Verification items for the finished model (mm, model axes). A direction names the side the tool comes from. Give positions to 0.01 mm unless a question says otherwise; leave off trailing zeros. Loops run counter-clockwise (first coordinate to the right, second up) from the corner with the lowest first, then second, coordinate; pieces in that order, holes last. Notation, with made-up numbers: (36.5, 41.5) - (55.5, 41.5) arc R25 ccw to (55.5, 65.5) - close; hole circle Ø8 at (22.25, -6). An arc over 180 degrees is marked (long way). Answer in a Markdown table with one row per item.
```python
from build123d import *

# Parameters (mm, degrees)
ESQUISSE1_R        = 1.6
BOSS_EXTRU_1_DEPTH = 1.6
ESQUISSE2_W        = 11
ESQUISSE2_H        = 9
BOSS_EXTRU_2_DEPTH = 12.7
ESQUISSE3_W        = 32.2
ESQUISSE3_H        = 9.1
BOSS_EXTRU_3_DEPTH = 14.9
ESQUISSE4_W        = 35.56
ESQUISSE4_H        = 17.78
BOSS_EXTRU_4_DEPTH = 12


with BuildPart() as part:
    # Esquisse1 → Boss.-Extru.1 (new body)
    with BuildSketch(Plane.XY):
        Polygon((0, 0), (100, 0), (100, -70), (30, -70), (0, -40), align=None)
        with Locations((3.5, -3.5)):
            Circle(ESQUISSE1_R, mode=Mode.SUBTRACT)
        with Locations((96.5, -3.5)):
            Circle(ESQUISSE1_R, mode=Mode.SUBTRACT)
        with Locations((3.5, -38.5)):
            Circle(ESQUISSE1_R, mode=Mode.SUBTRACT)
        with Locations((96.5, -66.5)):
            Circle(ESQUISSE1_R, mode=Mode.SUBTRACT)
    extrude(amount=BOSS_EXTRU_1_DEPTH)

    # Esquisse2 → Boss.-Extru.2 (add)
    with BuildSketch(Plane.XY.offset(1.6)):
        with Locations((14, -4.5)):
            Rectangle(ESQUISSE2_W, ESQUISSE2_H)
        with Locations((26, -4.5)):
            Rectangle(ESQUISSE2_W, ESQUISSE2_H)
        with Locations((38, -4.5)):
            Rectangle(ESQUISSE2_W, ESQUISSE2_H)
    extrude(amount=BOSS_EXTRU_2_DEPTH)

    # Esquisse3 → Boss.-Extru.3 (add)
    with BuildSketch(Plane.XY.offset(1.6)):
        with Locations((71.1, -4.55)):
            Rectangle(ESQUISSE3_W, ESQUISSE3_H)
    extrude(amount=BOSS_EXTRU_3_DEPTH)

    # Esquisse4 → Boss.-Extru.4 (add)
    with BuildSketch(Plane.XY.offset(1.6)):
        with Locations((65.28, -36.14)):
            Rectangle(ESQUISSE4_W, ESQUISSE4_H)
    extrude(amount=BOSS_EXTRU_4_DEPTH)


solid = part.part
```
Q1. Tool access check on faces 1 (the face through (87.2, -5, 9)), 2 (the face through (26, -9, 8)), 3 (the face through (55, -5, 9)). Record the directions out of +Z, -Z, +X, -X, +Y, -Y that give a thin tool (end or side, any length) a straight path to the whole face; none if there is none.
Completed:
| item | result |
|---|---|
| face 1 | +Z, +X, +Y, -Y |
| face 2 | +Z, -X, -Y |
| face 3 | +Z, +Y |
Q2. Go/stop test with flat-tipped pins: P1, Ø6, axis at y = -34.5, z = 11, coming from the +X side; P2, Ø7.5, axis at y = -6.5, z = 11, coming from the +X side; P3, Ø7, axis at y = -5, z = 8, coming from the -X side. Record where each tip stops, or that it passes through.
Completed:
| item | result |
|---|---|
| P1 | x = 83.06 |
| P2 | x = 87.2 |
| P3 | x = 8.5 |
Q3. Sectioned sample at A-A (y = -38.5). Record the cut outline in (x, z), and give its area (3 significant figures).
Completed:
| item | result |
|---|---|
| outline | (0, 0) - (1.9, 0) - (1.9, 1.6) - (0, 1.6) - close; (5.1, 0) - (100, 0) - (100, 1.6) - (83.06, 1.6) - (83.06, 13.6) - (47.5, 13.6) - (47.5, 1.6) - (5.1, 1.6) - close |
| area | 582 mm^2 |
Q4. Sectioned sample at D-D (y = -3.5). Record the cut outline in (x, z), and give its area (3 significant figures).
Completed:
| item | result |
|---|---|
| outline | (0, 0) - (1.9, 0) - (1.9, 1.6) - (0, 1.6) - close; (5.1, 0) - (94.9, 0) - (94.9, 1.6) - (87.2, 1.6) - (87.2, 16.5) - (55, 16.5) - (55, 1.6) - (43.5, 1.6) - (43.5, 14.3) - (32.5, 14.3) - (32.5, 1.6) - (31.5, 1.6) - (31.5, 14.3) - (20.5, 14.3) - (20.5, 1.6) - (19.5, 1.6) - (19.5, 14.3) - (8.5, 14.3) - (8.5, 1.6) - (5.1, 1.6) - close; (98.1, 0) - (100, 0) - (100, 1.6) - (98.1, 1.6) - close |
| area | 1,050 mm^2 |
Q5. Sectioned sample at B-B (z = 11.75). Record the cut outline in (x, y).
Completed:
| item | result |
|---|---|
| outline | (8.5, -9) - (19.5, -9) - (19.5, 0) - (8.5, 0) - close; (20.5, -9) - (31.5, -9) - (31.5, 0) - (20.5, 0) - close; (32.5, -9) - (43.5, -9) - (43.5, 0) - (32.5, 0) - close; (47.5, -45.03) - (83.06, -45.03) - (83.06, -27.25) - (47.5, -27.25) - close; (55, -9.1) - (87.2, -9.1) - (87.2, 0) - (55, 0) - close |
Q6. Draft check along Y on faces 4 (the face through (65, -45.03, 8)), 5 (the face through (47.5, -36, 8)), 6 (the face through (4.24, -39.92, 0.79)), 7 (the face through (49, 0, 1)). Enter one of: +Y half, -Y half, draft (parallel to the pull), parting line (faces both ways), or undercut.
Completed:
| item | result |
|---|---|
| face 4 | -Y half |
| face 5 | draft |
| face 6 | undercut |
| face 7 | +Y half |
Q7. Thickness scan on line 1 (Y direction, x = 96.5, z = 0.85); line 2 (X direction, y = -3, z = 8.25); line 3 (Y direction, x = 64.5, z = 2.5). Record the ranges inside material, lowest first.
Completed:
| item | result |
|---|---|
| line 1 | -70 to -68.1, -64.9 to -5.1, -1.9 to 0 |
| line 2 | 8.5 to 19.5, 20.5 to 31.5, 32.5 to 43.5, 55 to 87.2 |
| line 3 | -45.03 to -27.25, -9.1 to 0 |
Q8. Sectioned sample at C-C (x = 3.5). Record the cut outline in (y, z), and give its area (3 significant figures).
Completed:
| item | result |
|---|---|
| outline | (-43.5, 0) - (-40.1, 0) - (-40.1, 1.6) - (-43.5, 1.6) - close; (-36.9, 0) - (-5.1, 0) - (-5.1, 1.6) - (-36.9, 1.6) - close; (-1.9, 0) - (0, 0) - (0, 1.6) - (-1.9, 1.6) - close |
| area | 59.4 mm^2 |
